Verification items for the finished model (mm, model axes). A direction names the side the tool comes from. Round coordinates to 2 decimals unless told otherwise and drop trailing zeros. Write each loop counter-clockwise with the first axis right and the second up, starting at its lowest first coordinate (ties: lowest second). Pieces come first, ordered by that corner, then holes. Notation, with made-up numbers: (34.5, -35.75) -> (89.5, -35.75) arc R11 cw to (89.5, -22.75) -> close; hole circle Ø10 at (50, 63). An arc over 180 degrees is marked (long way). Answer as a JSON object with one key per item and string values. Group by question number.
(1) Sectioned sample at A-A on x = 25. Record the cut outline in (y, z).
(2) Set-up check for faces 4 (the face through (5.77, -23.91, 25.38)), 5 (the face through (60.28, -9.86, 44.566)): record each of +Z, -Z, +X, -X, +Y, -Y from which the full face is reachable in a straight line by a thin tool's end or side.
(3) Sectioned sample at B-B on y = -31. Record the cut outline in (x, z), and give its area (3 significant figures).
(4) Sectioned sample at D-D on y = -15. Record the cut outline in (x, z).
(5) Draft check along Z on faces 1 (the face through (74.716, -39.72, 19.366)), 2 (the face through (65.129, -32.988, 42.334)), 3 (the face through (6.503, -43.748, 22.375)). Enter one of: released by +Z, released by -Z, zero draft, split by the parting line, or undercut.
(6) Gauge pin test, flat ends, axial feed: pin 1 Ø1 at (y, z) = (-50.5, 7) entering from +X; pin 2 Ø2 at (y, z) = (-35, 7) entering from -X; pin 3 Ø6 at (x, y) = (58, -47.5) entering from +Z. Record the tip position at first contact, or that the pin passes through.
(7) Sectioned sample at C-C on z = 6.5. Record the cut outline in (x, y).
(8) Scan lines: L1, parallel to X at y = -30, z = 37; L2, parallel to X at y = -42, z = 23; L3, parallel to X at y = -56.5, z = 20.5. Record each from-to range of solid material in increasing order. Write a range as from..to.
```python
from build123d import *

# Parameters (mm, degrees)
F0_W        = 80
F0_H        = 50
F1_DEPTH    = 60
F2_T1_DEPTH = 14.4048552446
F2_T3_DEPTH = 287.737725616
F2_T5_DEPTH = 267.737725616
F2_T7_DEPTH = 257.737725616
F3_W        = 10
F3_H        = 20
F4_DEPTH    = 59.8932080195


# Not quite as in the source:
# - a fillet or chamfer that OpenCascade refuses, or shapes differently, is made with other operations: its cross-section is extruded or revolved along the edge and cut away or added


with BuildPart() as f1:
    # F0 (on Front) → F1 (new body)
    with BuildSketch(Plane.XZ):
        with Locations((40, 25)):
            Rectangle(F0_W, F0_H)
    extrude(amount=F1_DEPTH)

    # F2: chamfer of 40 x 10.7179676972 on 3 edges, made by hand

    # F2_s2 → F2_t1 (cut)
    with BuildSketch(Plane(origin=(15.4641016151, -4.1435935394, 57.7128129211), x_dir=(0.2588190451, 0.9659258263, 0), z_dir=(0.2581988897, -0.069184184, 0.963611375))):
        Polygon((1.3870070824, -68.9498200994), (-8.9657547217, -28.8537460449), (-40.024040134, -68.9498200994), align=None)
    extrude(amount=F2_T1_DEPTH, mode=Mode.SUBTRACT)

    # F2_s4 → F2_t3 (cut)
    with BuildSketch(Plane.YZ.offset(-103.868862808)):
        Polygon((-20, 50), (-60, 39.2820323028), (-60, 50), align=None)
    extrude(amount=F2_T3_DEPTH, mode=Mode.SUBTRACT)

    # F2_s6 → F2_t5 (cut)
    with BuildSketch(Plane.XZ.offset(-103.868862808)):
        Polygon((80, 39.2820323028), (40, 50), (80, 50), align=None)
    extrude(amount=F2_T5_DEPTH, mode=Mode.SUBTRACT)

    # F2_s8 → F2_t7 (cut)
    with BuildSketch(Plane.XY.offset(-103.868862808)):
        Polygon((80, -20), (69.2820323028, -60), (80, -60), align=None)
    extrude(amount=F2_T7_DEPTH, mode=Mode.SUBTRACT)

    # F3 (on face) → F4 (cut, through all)
    with BuildSketch(Plane(origin=(15.4641016151, -4.1435935394, 57.7128129211), x_dir=(0.9660917831, 0.0184902509, -0.2575359728), z_dir=(0.2581988897, -0.069184184, 0.963611375))):
        with Locations((-1.3299316186, -32.0328700794)):
            Rectangle(F3_W, F3_H)
    extrude(amount=-F4_DEPTH, mode=Mode.SUBTRACT)


solid = f1.part
```
Computed values:
{
 "1": {"outline": "(-60, 0) -> (0, 0) -> (0, 50) -> (-20, 50) -> (-60, 39.28) -> close"},
 "2": {"face 4": "none", "face 5": "+Z, +X, +Y, -Y"},
 "3": {"outline": "(0, 22.35) -> (6.58, 47.05) -> (0, 47.05) -> close; (4.39, 0) -> (77.05, 0) -> (77.05, 39.28) -> (48.05, 47.05) -> (16.94, 47.05) -> close", "area": "3,090 mm2"},
 "4": {"outline": "(0, 0) -> (80, 0) -> (80, 39.28) -> (40, 50) -> (0, 50) -> close"},
 "5": {"face 1": "zero draft", "face 2": "released by +Z", "face 3": "undercut"},
 "6": {"pin 1": "x = 71.96", "pin 2": "x = 6.07", "pin 3": "z = 43.44"},
 "7": {"outline": "(0, -60) -> (69.28, -60) -> (80, -20) -> (80, 0) -> (0, 0) -> (0, -22.56) -> (5.96, -22.56) -> (6.35, -42.61) -> (0, -42.61) -> close"},
 "8": {"L1": "0..3.89, 14.24..77.32", "L2": "0..0.38, 10.73..74.11", "L3": "0..70.22"}
}
